Here's how the part is built. I have some questions about the finished solid (model axes, mm). Face numbers are marked on the shaded views. A direction names the side the tool comes from. Round coordinates to 2 decimals unless told otherwise and drop trailing zeros. Loops run counter-clockwise (first coordinate to the right, second up) from the corner with the lowest first, then second, coordinate; pieces in that order, holes last. Notation, with made-up numbers: (80, -18.75) - (130, -18.75) arc R17 ccw to (130, 0.25) - close; hole circle Ø7 at (-23, 27). An arc over 180 degrees is marked (long way). Answer as a JSON object with one key per item and string values. Group by question number.
1) I want a section at A-A, the plane y = 19. Please give me the cut outline in (x, z), then the cut area to 3 significant figures.
2) I want a section at D-D, the plane x = 37. Please give me the cut outline in (y, z).
3) Which directions (+Z, -Z, +X, -X, +Y, -Y) give clear straight access to the entire face, cutting with the end or side of a thin tool? Please do the marked faces 1, 2 and 3.
4) If I drill on line 1 along Y through (x, z) = (43, -23.5); line 2 along Y through (x, z) = (18, -13.5); line 3 along Z through (x, y) = (40, 27.5), over which ranges is the centre line in solid material (lowest first)? Write a range as [from, to].
5) If we mould it in two halves opening along Y, with no side actions, what happens to the marked faces 4, 5 and 6? For each: pulls with the +Y half, pulls with the -Y half, needs draft (parallel to the pull), parting line crosses it, or undercut.
6) Will these pins go through, and if not, where does the flat tip stop? P1, Ø1.2, axis at x = 44, z = -14, coming from the +Y side; P2, Ø3, axis at x = 39, z = 27, coming from the -Y side; P3, Ø6, axis at y = 19, z = 5.5, coming from the +X side.
7) I want a section at B-B, the plane x = 18. Please give me the cut outline in (y, z), then the cut area to 3 significant figures.
8) I want a section at C-C, the plane z = -28. Please give me the cut outline in (x, y), then the cut area to 3 significant figures.
from build123d import *

# Parameters (mm, degrees)
SKETCH1_W           = 36
SKETCH1_H           = 38
BOSS_EXTRUDE1_DEPTH = 33
SKETCH2_R           = 12
CUT_EXTRUDE1_DEPTH  = 85.237758755
SKETCH3_W           = 20
SKETCH3_H           = 26
BOSS_EXTRUDE2_DEPTH = 10
SKETCH7_R           = 9
CUT_EXTRUDE4_DEPTH  = 5
CUT_EXTRUDE5_DEPTH  = 89.971905678


with BuildPart() as part:
    # Sketch1 → Boss-Extrude1 (new, symmetric)
    with BuildSketch(Plane.XY):
        with Locations((18, 19)):
            Rectangle(SKETCH1_W, SKETCH1_H)
    extrude(amount=BOSS_EXTRUDE1_DEPTH, both=True)

    # Sketch2 → Cut-Extrude1 (cut, through all)
    with BuildSketch(Plane.XY.offset(33)):
        with Locations((18, 19)):
            Circle(SKETCH2_R)
    extrude(amount=-CUT_EXTRUDE1_DEPTH, mode=Mode.SUBTRACT)

    # Sketch3 → Boss-Extrude2 (add)
    with BuildSketch(Plane(origin=(36, 0, 0), x_dir=(0, 0, -1), z_dir=(1, 0, 0))):
        with Locations((-23, 19)):
            Rectangle(SKETCH3_W, SKETCH3_H)
        with Locations((23, 19)):
            Rectangle(SKETCH3_W, SKETCH3_H)
    extrude(amount=BOSS_EXTRUDE2_DEPTH)

    # Sketch7 → Cut-Extrude4 (cut)
    with BuildSketch(Plane(origin=(46, 0, 0), x_dir=(0, 0, -1), z_dir=(1, 0, 0))):
        with Locations(Location((-23, 19, 0), (0, 0, 90))):
            Circle(SKETCH7_R)
        with Locations(Location((23, 19, 0), (0, 0, 90))):
            Circle(SKETCH7_R)
    extrude(amount=-CUT_EXTRUDE4_DEPTH, mode=Mode.SUBTRACT)

    # Sketch8 → Cut-Extrude5 (cut, through all)
    with BuildSketch(Plane.XY.offset(33)):
        Polygon((46, 19), (46, 22), (41, 22), (41, 16), (46, 16), align=None)
    extrude(amount=-CUT_EXTRUDE5_DEPTH, mode=Mode.SUBTRACT)


solid = part.part
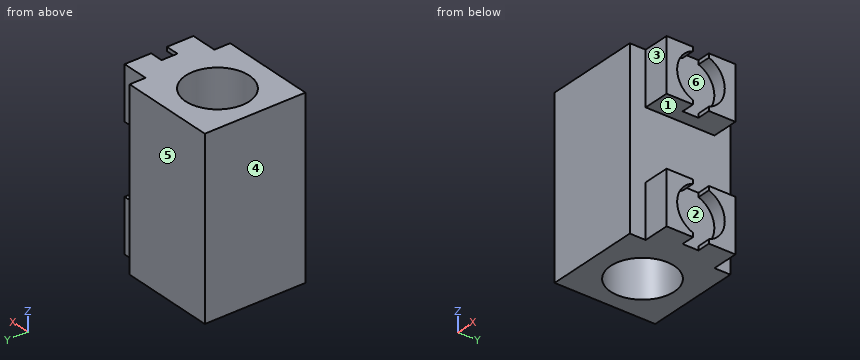
Outcome:
{
 "1": {"outline": "(0, -33) - (6, -33) - (6, 33) - (0, 33) - close; (30, -33) - (41, -33) - (41, -13) - (36, -13) - (36, 13) - (41, 13) - (41, 33) - (30, 33) - close", "area": "992 mm^2"},
 "2": {"outline": "(6, -33) - (32, -33) - (32, -13) - (6, -13) - close; (6, 13) - (32, 13) - (32, 33) - (6, 33) - close"},
 "3": {"face 1": "+X, +Y, -Y", "face 2": "+X", "face 3": "+Z, -Z, +X, -Y"},
 "4": {"line 1": "[6, 10.01], [27.99, 32]", "line 2": "[0, 7], [31, 38]", "line 3": "[-33, -13], [13, 33]"},
 "5": {"face 4": "needs draft", "face 5": "pulls with the +Y half", "face 6": "undercut"},
 "6": {"P1": "y = 32", "P2": "y = 6", "P3": "x = 36"},
 "7": {"outline": "(0, -33) - (7, -33) - (7, 33) - (0, 33) - close; (31, -33) - (38, -33) - (38, 33) - (31, 33) - close", "area": "924 mm^2"},
 "8": {"outline": "(0, 0) - (36, 0) - (36, 6) - (46, 6) - (46, 11.52) - (41, 11.52) - (41, 26.48) - (46, 26.48) - (46, 32) - (36, 32) - (36, 38) - (0, 38) - close; hole circle Ø24 at (18, 19)", "area": "1,100 mm^2"}
}
